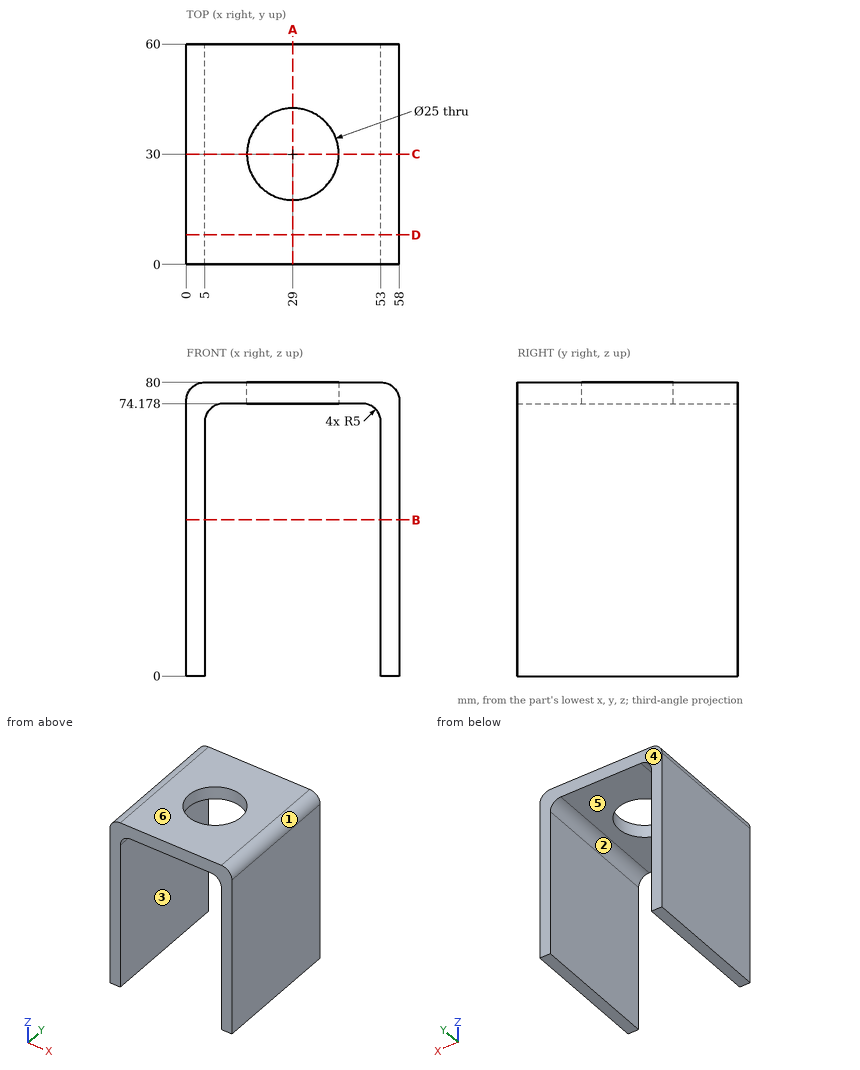
Could you check a few things on this drawing? It's one solid part, dimensions in mm from its lowest x, y, z. A direction names the side the tool comes from. Coordinates: 2 decimals unless noted, no trailing zeros. Order: outer loops, then holes, each group sorted by start corner. A loop starts at its lowest first (then second) coordinate and runs counter-clockwise, first axis right, second up.
1) I need wall thicknesses on line 1 (Y direction, x = 29, z = 76.55); line 2 (X direction, y = 38.5, z = 5); line 3 (Z direction, x = 23.5, y = 51). Which ranges of each line are inside material? Lowest first, please.
2) Imagine slicing it at D-D on y = 8. List the corners of the cut face in (x, z) for me, and give its area (3 significant figures).
3) Which directions (+Z, -Z, +X, -X, +Y, -Y) give clear straight access to the entire face, cutting with the end or side of a thin tool? Please do the marked faces 5 and 6.
4) Imagine slicing it at B-B on z = 42.5. List the corners of the cut face in (x, y) for me, and give its area (3 significant figures).
5) We'd pull the mould along X, two halves only. Please class the marked faces 1, 2, 3 and 4: +X half, -X half, draft (parallel to the pull), parting line (faces both ways), or undercut.
6) Will these pins go through, and if not, where does the flat tip stop? pin 1 (22.5 mm diameter, centred on x = 29, y = 30, fed in from -Z); pin 2 (8 mm diameter, centred on x = 43.5, y = 10, fed in from -Z).
7) Imagine slicing it at C-C on y = 30. List the corners of the cut face in (x, z) for me.
8) Imagine slicing it at A-A on x = 29. List the corners of the cut face in (y, z) for me, and give its area (3 significant figures).
Response values:
1. line 1: y = 0 to 17.5, 42.5 to 60
1. line 2: x = 0 to 5, 53 to 58
1. line 3: z = 74.18 to 80
2. outline: (0, 0) - (5, 0) - (5, 69.18) arc R5 cw to (10, 74.18) - (48, 74.18) arc R5 cw to (53, 69.18) - (53, 0) - (58, 0) - (58, 75) arc R5 ccw to (53, 80) - (5, 80) arc R5 ccw to (0, 75) - close
2. area: 1,080 mm2
3. face 5: -Z, +Y, -Y
3. face 6: +Z, +X, -X, +Y, -Y
4. outline: (0, 0) - (5, 0) - (5, 60) - (0, 60) - close; (53, 0) - (58, 0) - (58, 60) - (53, 60) - close
4. area: 600 mm2
5. face 1: +X half
5. face 2: undercut
5. face 3: undercut
5. face 4: draft
6. pin 1: passes through
6. pin 2: stops at z = 74.18
7. outline: (0, 0) - (5, 0) - (5, 69.18) arc R5 cw to (10, 74.18) - (16.5, 74.18) - (16.5, 80) - (5, 80) arc R5 ccw to (0, 75) - close; (41.5, 74.18) - (48, 74.18) arc R5 cw to (53, 69.18) - (53, 0) - (58, 0) - (58, 75) arc R5 ccw to (53, 80) - (41.5, 80) - close
8. outline: (0, 74.18) - (17.5, 74.18) - (17.5, 80) - (0, 80) - close; (42.5, 74.18) - (60, 74.18) - (60, 80) - (42.5, 80) - close
8. area: 204 mm2
